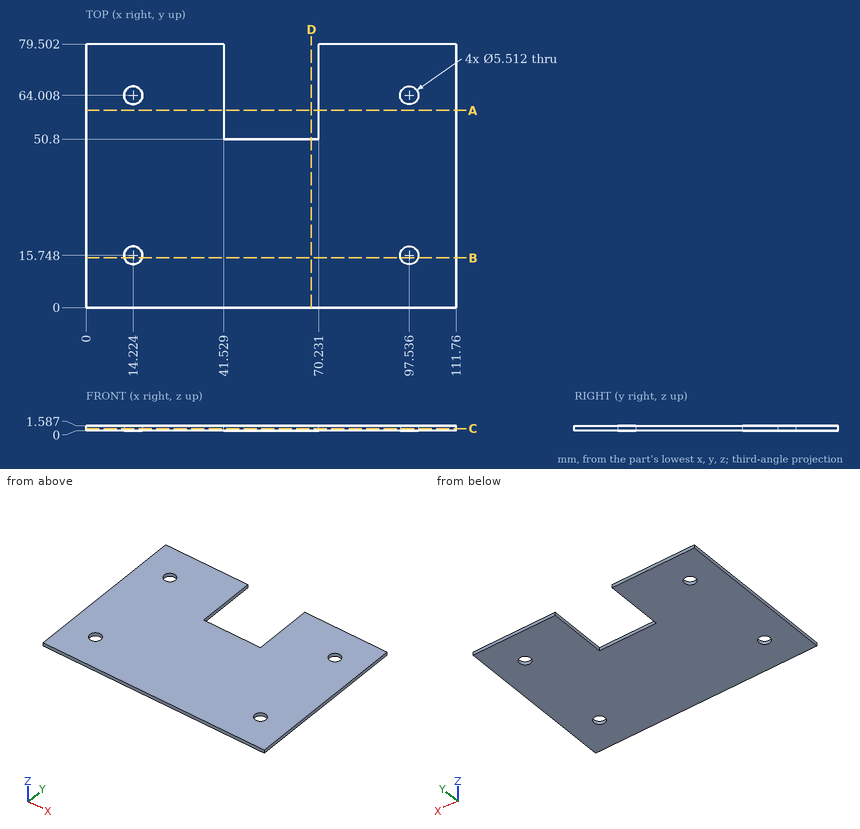
For this review, use the dimensioned drawing (mm, ordinates from the lowest corner) and the shaded views. Give positions to 0.01 mm unless a question says otherwise; leave off trailing zeros. Loops run counter-clockwise (first coordinate to the right, second up) from the corner with the lowest first, then second, coordinate; pieces in that order, holes last.
Item 1: Take a section at B-B, the plane y = 15. State the section outline as (x, z) points.
Item 2: Take a section at D-D, the plane x = 68. State the section outline as (y, z) points.
Item 3: Take a section at C-C, the plane z = 0.65. State the section outline as (x, y) points (1 decimal), and give its area (3 significant figures).
Item 4: Insertion check: pin 1 (5 mm diameter, centred on x = 14.224, y = 15.748, fed in from +Z). The pin has a flat end and moves straight along its axis. Give the tip position at first contact, or say it passes through.
Item 5: Take a section at A-A, the plane y = 59.5. State the section outline as (x, z) points, and give its area (3 significant figures).
Item 6: For line 1 along Y through (x, z) = (98.5, 1.3) (1 decimal); line 2 along Y through (x, z) = (43.5, 1.2); line 3 along X through (y, z) = (63, 0.2), list the stretches that pass through material, from the lowest coordinate up.
Calculated:
1. outline: (0, 0) - (11.57, 0) - (11.57, 1.59) - (0, 1.59) - close; (16.88, 0) - (94.88, 0) - (94.88, 1.59) - (16.88, 1.59) - close; (100.19, 0) - (111.76, 0) - (111.76, 1.59) - (100.19, 1.59) - close
2. outline: (0, 0) - (50.8, 0) - (50.8, 1.59) - (0, 1.59) - close
3. outline: (0, 0) - (111.8, 0) - (111.8, 79.5) - (70.2, 79.5) - (70.2, 50.8) - (41.5, 50.8) - (41.5, 79.5) - (0, 79.5) - close; hole circle Ø5.5 at (14.2, 15.7); hole circle Ø5.5 at (14.2, 64); hole circle Ø5.5 at (97.5, 15.7); hole circle Ø5.5 at (97.5, 64)
3. area: 7,970 mm2
4. pin 1: passes through
5. outline: (0, 0) - (41.53, 0) - (41.53, 1.59) - (0, 1.59) - close; (70.23, 0) - (111.76, 0) - (111.76, 1.59) - (70.23, 1.59) - close
5. area: 132 mm2
6. line 1: y = 0 to 13.2, 18.3 to 61.4, 66.6 to 79.5
6. line 2: y = 0 to 50.8
6. line 3: x = 0 to 11.66, 16.79 to 41.53, 70.23 to 94.97, 100.1 to 111.76
